from build123d import *

# Parameters (mm, degrees)
SKETCH1_R           = 50
SKETCH1_R_2         = 15
BOSS_EXTRUDE1_DEPTH = 40
SKETCH2_W           = 20
SKETCH2_H           = 5


with BuildPart() as part:
    # Sketch1 → Boss-Extrude1 (new body)
    with BuildSketch(Plane.XY):
        Circle(SKETCH1_R)
        Circle(SKETCH1_R_2, mode=Mode.SUBTRACT)
    extrude(amount=BOSS_EXTRUDE1_DEPTH)

    # Sketch2 → Cut-Revolve1 (revolve, cut)
    with BuildSketch(Plane(origin=(0, 0, 0), x_dir=(0, 0, -1), z_dir=(1, 0, 0)), mode=Mode.PRIVATE) as cut_revolve1_sk:
        with Locations((-20, 47.5)):
            Rectangle(SKETCH2_W, SKETCH2_H)
        with Locations((-20, -47.5)):
            Rectangle(SKETCH2_W, SKETCH2_H)
    revolve(cut_revolve1_sk.sketch.rotate(Axis((0, 0, -46.879295237), (0, 0, 1)), 90), axis=Axis((0, 0, -46.879295237), (0, 0, 1)), mode=Mode.SUBTRACT)


solid = part.part
For this review, take the finished solid that the model builds, in its own axes (mm). A direction names the side the tool comes from. Round coordinates to 2 decimals unless told otherwise and drop trailing zeros. Write each loop counter-clockwise with the first axis right and the second up, starting at its lowest first coordinate (ties: lowest second). Pieces come first, ordered by that corner, then holes. Notation, with made-up numbers: (1, 2.25) -> (50, 2.25) arc R9 cw to (50, 17.25) -> close; hole circle Ø1 at (70.25, 44). An arc over 180 degrees is marked (long way). Use CSV: the item, a comma, the result in double quotes.
(1) To check wall thickness, follow L1, parallel to Y at x = 0, z = 19; L2, parallel to Z at x = 30, y = 37; L3, parallel to Y at x = -0.5, z = 4. State the ranges of each line that lie inside material, in increasing order. Write a range as [from, to].
Computed values:
L1,"[-45, -15], [15, 45]"
L2,"[0, 10], [30, 40]"
L3,"[-50, -14.99], [14.99, 50]"
(2) Consider section C-C, the plane z = 3. Give the boundary of the cut face in (x, y).
Computed values:
outline,"circle Ø100 at (0, 0); hole circle Ø30 at (0, 0)"
(3) Consider section D-D, the plane y = -24. Give the boundary of the cut face in (x, z), plus the area to 3 significant figures.
Computed values:
outline,"(-43.86, 0) -> (43.86, 0) -> (43.86, 10) -> (38.07, 10) -> (38.07, 30) -> (43.86, 30) -> (43.86, 40) -> (-43.86, 40) -> (-43.86, 30) -> (-38.07, 30) -> (-38.07, 10) -> (-43.86, 10) -> close"
area,"3,280 mm²"
(4) Draft analysis for pull direction Z (two halves, no side actions). For faces 3 (the face through (-20.765, 39.923, 19.86)), 4 (the face through (-12, -10, 0)), 5 (the face through (-41, -19, 30)), 6 (the face through (47.69, 15.02, 34.93)), state which applies: +Z half, -Z half, draft (parallel to the pull), parting line (faces both ways), or undercut.
Computed values:
face 3,"undercut"
face 4,"-Z half"
face 5,"undercut"
face 6,"draft"
(5) For faces 1 (the face through (-41, -19, 10)), 2 (the face through (-12, -10, 40)), list the 3-axis set-ups (+Z, -Z, +X, -X, +Y, -Y) from which the entire face can be reached by the end or side of a thin tool; tool diameter is ignored.
Computed values:
face 1,"none"
face 2,"+Z, +X, -X, +Y, -Y"
(6) Consider section A-A, the plane x = 0. Give the boundary of the cut face in (y, z).
Computed values:
outline,"(-50, 0) -> (-15, 0) -> (-15, 40) -> (-50, 40) -> (-50, 30) -> (-45, 30) -> (-45, 10) -> (-50, 10) -> close; (15, 0) -> (50, 0) -> (50, 10) -> (45, 10) -> (45, 30) -> (50, 30) -> (50, 40) -> (15, 40) -> close"
(7) Clearance check with flat-ended pins moving along their axes: P1, Ø3, axis at y = 23.5, z = 34, coming from the -X side; P2, Ø6, axis at y = 32, z = 19, coming from the -X side; P3, Ø6, axis at y = -10.5, z = 30, coming from the +X side. State where each tip first meets the part, or that it passes through.
Computed values:
P1,"x = -44.9"
P2,"x = -34.41"
P3,"x = 49.43"
